from build123d import *
from build123d.topology import SkipClean

# Parameters (mm, degrees)
BOSS_EXTRU_1_START      = -6
BOSS_EXTRU_1_DEPTH      = 6
BOSS_EXTRU_2_START      = -6
BOSS_EXTRU_2_DEPTH      = 2
ENL_V_START             = -4
ESQUISSE3_5_R           = 2.55
ENL_V_MAT_EXTRU_1_DEPTH = 4
ENL_V_START_2           = -16.5
ENL_V_MAT_EXTRU_5_DEPTH = 10.5
CONG_1_R                = 2
CHANFREIN1_SIZE         = 0.5
SYM_TRIE1_START         = -2
SYM_TRIE1_DEPTH         = 10.5
SYM_TRIE1_START_2       = -8
SYM_TRIE1_2_DEPTH       = 4
SYM_TRIE1_START_3       = -7.5000001
SYM_TRIE1_3_DEPTH       = 5.5000001
SYM_TRIE1_START_4       = -4
SYM_TRIE1_4_DEPTH       = 2
SYM_TRIE1_7_DEPTH       = 0.4999999
M3_CLEARANCE_HOLE1_D    = 3.4
BOSS_EXTRU_3_DEPTH      = 8.5
ENL_V_START_3           = -8.5
ENL_V_MAT_EXTRU_2_DEPTH = 8.5
ENL_V_START_4           = -6.5
ESQUISSE5_R             = 1.125
ENL_V_MAT_EXTRU_3_DEPTH = 6
ESQUISSE5_3_R           = 1.125
ENL_V_MAT_EXTRU_4_DEPTH = 6.5
CONG_2_R                = 0.5
CONG_3_R                = 1.5
ENL_V_START_5           = -7.5
ESQUISSE9_R             = 4
ENL_V_MAT_EXTRU_8_DEPTH = 7.5
CONG_5_R                = 1.5


with BuildPart() as part:
    # Esquisse1 → Révolution1 (revolve)
    with BuildSketch(Plane.XY):
        Polygon((-8.5, 8.5), (-6, 8.5), (-6, 0), (-3.5, 0), (-3.5, -1), (-4.383974596, -1), (-5.25, -1.5), (-6.5, -1.5), (-6.5, -6.5), (-6.8, -6.5), (-6.8, -7.2), (-6.5, -7.2), (-6.5, -8), (-8.5, -8), align=None)
    revolve(axis=Axis((0, 6.43509573, 0), (0, -1, 0)))

    # Esquisse3 → Boss.-Extru.1 (add)
    with BuildSketch(Plane.XZ.offset(8).offset(BOSS_EXTRU_1_START)):
        with BuildLine():
            ThreePointArc((-7.928571429, 3.06394437), (-7.728470361, 3.5384666), (-7.5, 4))
            Line((-7.5, 4), (-10.5, 4))
            ThreePointArc((-10.5, 4), (-14.5, 0), (-10.5, -4))
            Line((-10.5, -4), (-7.5, -4))
            ThreePointArc((-7.5, -4), (-7.728470361, -3.5384666), (-7.928571429, -3.06394437))
            ThreePointArc((-7.928571429, -3.06394437), (-8.196108254, -2.252511816), (-8.380833333, -1.418320358))
            ThreePointArc((-8.380833333, -1.418320358), (-13.05, 0), (-8.380833333, 1.418320358))
            ThreePointArc((-8.380833333, 1.418320358), (-8.196108254, 2.252511816), (-7.928571429, 3.06394437))
        make_face()
    extrude(amount=BOSS_EXTRU_1_DEPTH)

    # Esquisse3<4> → Boss.-Extru.2 (add)
    with BuildSketch(Plane.XZ.offset(8).offset(BOSS_EXTRU_2_START)):
        with BuildLine():
            ThreePointArc((-8.380833333, -1.418320358), (-8.5, 0), (-8.380833333, 1.418320358))
            ThreePointArc((-8.380833333, 1.418320358), (-13.05, 0), (-8.380833333, -1.418320358))
        make_face()
    extrude(amount=BOSS_EXTRU_2_DEPTH)

    # Esquisse3<5> → Enlèv. mat.-Extru.1 (cut)
    with BuildSketch(Plane.XZ.offset(8).offset(ENL_V_START)):
        with Locations((-10.5, 0)):
            Circle(ESQUISSE3_5_R)
    extrude(amount=ENL_V_MAT_EXTRU_1_DEPTH, mode=Mode.SUBTRACT)

    # Esquisse3<7> → Enlèv. mat.-Extru.5 (cut)
    with BuildSketch(Plane.XZ.offset(8).offset(ENL_V_START_2)):
        with BuildLine():
            ThreePointArc((-7.5, 4), (-8.5, 0), (-7.5, -4))
            Line((-7.5, -4), (-7.5, 4))
        make_face()
    extrude(amount=ENL_V_MAT_EXTRU_5_DEPTH, mode=Mode.SUBTRACT)

    # Congé1
    cong_1_edges = [part.edges().sort_by_distance(p)[0] for p in [
        (-7.5, -5, 4),
        (-7.5, -5, -4),
    ]]
    fillet(cong_1_edges, radius=CONG_1_R)

    # Chanfrein1
    chanfrein1_edges = [part.edges().sort_by_distance(p)[0] for p in [
        (-8.06008453, -8, 0.741156191),
    ]]
    chamfer(chanfrein1_edges, length=CHANFREIN1_SIZE)

    # Symétrie1: read off the stored shape, not the designer's step
    # Symétrie1 outline → Symétrie1 (cut)
    with BuildSketch(Plane(origin=(0, 0, 0), x_dir=(1, 0, 0), z_dir=(0, 1, 0)).offset(SYM_TRIE1_START)):
        with BuildLine():
            Line((7.5, 4), (7.5, -4))
            ThreePointArc((7.5, -4), (8.5, 0), (7.5, 4))
        make_face()
    extrude(amount=SYM_TRIE1_DEPTH, mode=Mode.SUBTRACT)

    # Sym_trie1 2 outline → Sym_trie1 2 (cut)
    with BuildSketch(Plane(origin=(0, 0, 0), x_dir=(1, 0, 0), z_dir=(0, 1, 0)).offset(SYM_TRIE1_START_2)):
        with BuildLine():
            ThreePointArc((8.380833333, 1.418320358), (7.95, 0), (8.380833333, -1.418320358))
            ThreePointArc((8.380833333, -1.418320358), (8.5, 0), (8.380833333, 1.418320358))
        make_face()
    extrude(amount=SYM_TRIE1_2_DEPTH, mode=Mode.SUBTRACT)

    # Sym_trie1 3 outline → Sym_trie1 3 (add)
    with BuildSketch(Plane(origin=(0, 0, 0), x_dir=(1, 0, 0), z_dir=(0, 1, 0)).offset(SYM_TRIE1_START_3)):
        with BuildLine():
            ThreePointArc((6.975540357, -4.857142857), (7.69102387, -4.227189479), (8.61684397, -4))
            Line((8.61684397, -4), (10.5, -4))
            ThreePointArc((10.5, -4), (14.5, 0), (10.5, 4))
            Line((10.5, 4), (8.61684397, 4))
            ThreePointArc((8.61684397, 4), (7.69102387, 4.227189479), (6.975540357, 4.857142857))
            ThreePointArc((6.975540357, 4.857142857), (7.868349781, 3.215442696), (8.380833333, 1.418320358))
            ThreePointArc((8.380833333, 1.418320358), (13.05, 0), (8.380833333, -1.418320358))
            ThreePointArc((8.380833333, -1.418320358), (7.868349781, -3.215442696), (6.975540357, -4.857142857))
        make_face()
    extrude(amount=SYM_TRIE1_3_DEPTH)

    # Sym_trie1 4 outline → Sym_trie1 4 (add)
    with BuildSketch(Plane(origin=(0, 0, 0), x_dir=(1, 0, 0), z_dir=(0, 1, 0)).offset(SYM_TRIE1_START_4)):
        with BuildLine():
            ThreePointArc((8.380833333, 1.418320358), (8.5, 0), (8.380833333, -1.418320358))
            ThreePointArc((8.380833333, -1.418320358), (13.05, 0), (8.380833333, 1.418320358))
        make_face()
    extrude(amount=SYM_TRIE1_4_DEPTH)

    # Sym_trie1 5 outline → Sym_trie1 5 (revolve, cut)
    with BuildSketch(Plane(origin=(10.5, 0, 0), x_dir=(1, 0, 0), z_dir=(0, 0, 1))):
        Polygon((3.05, -8), (2.55, -7.5), (2.55, -8), align=None)
    revolve(axis=Axis((10.5, 0, 0), (0, 1, 0)), mode=Mode.SUBTRACT)

    # Sym_trie1 6 outline → Sym_trie1 6 (revolve)
    with SkipClean():  # the faces are left unmerged after this step: merging them gives an invalid solid
        with BuildSketch(Plane(origin=(10.5, 0, 0), x_dir=(1, 0, 0), z_dir=(0, 0, 1))):
            Polygon((3.05, -7.5), (2.55, -7.5), (3.05, -8), align=None)
        revolve(axis=Axis((10.5, 0, 0), (0, 1, 0)))

    # Sym_trie1 7 outline → Sym_trie1 7 (add)
    with BuildSketch(Plane(origin=(0, 0, 0), x_dir=(1, 0, 0), z_dir=(0, 1, 0)).offset(SYM_TRIE1_START_2)):
        with BuildLine():
            ThreePointArc((8.2475, 2.056390953), (13.55, 0), (8.2475, -2.056390953))
            ThreePointArc((8.2475, -2.056390953), (7.933495012, -3.051173035), (7.5, -4))
            ThreePointArc((7.5, -4), (7.250447615, -4.436328367), (6.975540357, -4.857142857))
            ThreePointArc((6.975540357, -4.857142857), (7.69102387, -4.227189479), (8.61684397, -4))
            Line((8.61684397, -4), (10.5, -4))
            ThreePointArc((10.5, -4), (14.5, 0), (10.5, 4))
            Line((10.5, 4), (8.61684397, 4))
            ThreePointArc((8.61684397, 4), (7.69102387, 4.227189479), (6.975540357, 4.857142857))
            ThreePointArc((6.975540357, 4.857142857), (7.250447615, 4.436328367), (7.5, 4))
            ThreePointArc((7.5, 4), (7.933495012, 3.051173035), (8.2475, 2.056390953))
        make_face()
    extrude(amount=SYM_TRIE1_7_DEPTH)

    # M3 Clearance Hole1 (through all)
    with Locations(Plane(origin=(0, -4, 0), x_dir=(-1, 0, 0), z_dir=(0, -1, 0))):
        with Locations((10.5, 0), (-10.5, 0)):
            Hole(M3_CLEARANCE_HOLE1_D / 2)

    # Esquisse4 → Boss.-Extru.3 (add)
    with BuildSketch(Plane(origin=(0, 8.5, 0), x_dir=(1, 0, 0), z_dir=(0, 1, 0))):
        with BuildLine():
            Line((7.5, 14.5), (-7.5, 14.5))
            Line((-7.5, 14.5), (-7.5, 4))
            ThreePointArc((-7.5, 4), (-1.593272922, 8.349340177), (5.5, 6.480740698))
            Line((5.5, 6.480740698), (5.5, 13))
            Line((5.5, 13), (6, 13))
            Line((6, 13), (6, 6.020797289))
            ThreePointArc((6, 6.020797289), (6.825203691, 5.066220937), (7.5, 4))
            Line((7.5, 4), (7.5, 14.5))
        make_face()
    extrude(amount=-BOSS_EXTRU_3_DEPTH)

    # Esquisse4<3> → Enlèv. mat.-Extru.2 (cut)
    with BuildSketch(Plane(origin=(0, 8.5, 0), x_dir=(1, 0, 0), z_dir=(0, 1, 0)).offset(ENL_V_START_3)):
        with BuildLine():
            Line((6, 0), (6, 13))
            Line((6, 13), (5.5, 13))
            Line((5.5, 13), (5.5, 2.397915762))
            ThreePointArc((5.5, 2.397915762), (5.873670062, 1.224744871), (6, 0))
        make_face()
    extrude(amount=ENL_V_MAT_EXTRU_2_DEPTH, mode=Mode.SUBTRACT)

    # Esquisse5 → Enlèv. mat.-Extru.3 (cut)
    with BuildSketch(Plane(origin=(7.5, 0, 0), x_dir=(0, 0, -1), z_dir=(1, 0, 0)).offset(ENL_V_START_4)):
        with Locations((9.875, 4.2554)):
            Circle(ESQUISSE5_R)
        with BuildLine():
            Line((8.75, 8.5), (8.75, 4.2554))
            ThreePointArc((8.75, 4.2554), (9.875, 5.3804), (11, 4.2554))
            Line((11, 4.2554), (11, 8.5))
            Line((11, 8.5), (8.75, 8.5))
        make_face()
    extrude(amount=-ENL_V_MAT_EXTRU_3_DEPTH, mode=Mode.SUBTRACT)

    # Esquisse5<3> → Enlèv. mat.-Extru.4 (cut)
    with BuildSketch(Plane(origin=(7.5, 0, 0), x_dir=(0, 0, -1), z_dir=(1, 0, 0))):
        with Locations(Location((9.875, 4.2554, 0), (0, 0, 180))):
            Circle(ESQUISSE5_3_R)
    extrude(amount=-ENL_V_MAT_EXTRU_4_DEPTH, mode=Mode.SUBTRACT)

    # Congé2
    # the kernel refuses this fillet: 0.5 mm, written as the material it takes off along each edge
    with BuildSketch(Plane(origin=(5.5, 0, -2.397915762), x_dir=(0, 0, -1), z_dir=(0, 1, 0))) as cong_2_piece_1:
        with BuildLine():
            CenterArc((1.75539617, 0.5), CONG_2_R, 129.715137232, 140.284862768)
            ThreePointArc((1.435910637, 0.884615385), (0.749192225, 0.391603841), (0, 0))
            Line((0, 0), (1.75539617, 0))
        make_face()
    extrude(amount=12.888490425, mode=Mode.SUBTRACT)

    # Congé3
    cong_3_edges = [part.edges().sort_by_distance(p)[0] for p in [
        (7.5, 3.25, 4),
        (7.5, 4.25, -14.5),
        (-7.5, 4.25, -14.5),
        (-7.5, 3.25, 4),
    ]]
    fillet(cong_3_edges, radius=CONG_3_R)

    # Esquisse9 → Enlèv. mat.-Extru.8 (cut)
    with BuildSketch(Plane(origin=(0, 8.5, 0), x_dir=(1, 0, 0), z_dir=(0, 1, 0)).offset(ENL_V_START_5)):
        with Locations((-10.5, 0)):
            Circle(ESQUISSE9_R)
        with Locations((10.5, 0)):
            Circle(ESQUISSE9_R)
    extrude(amount=ENL_V_MAT_EXTRU_8_DEPTH, mode=Mode.SUBTRACT)

    # Congé5
    cong_5_edges = [part.edges().sort_by_distance(p)[0] for p in [
        (7.5, 4.75, -2.645751311),
        (7.5, 4.75, 2.645751311),
        (-7.5, 4.75, -2.645751311),
        (-7.5, 4.75, 2.645751311),
    ]]
    fillet(cong_5_edges, radius=CONG_5_R)


solid = part.part
Read the model definition and answer for the solid it produces. Units are mm, in the model's axes. A direction names the side the tool comes from. Give positions to 0.01 mm unless a question says otherwise; leave off trailing zeros. Loops run counter-clockwise (first coordinate to the right, second up) from the corner with the lowest first, then second, coordinate; pieces in that order, holes last. Notation, with made-up numbers: M -6,84 L 25,84 A17 ccw 25,104 Z; hole C -6.75,14 d5. An arc over 180 degrees is marked long. Write each question's results on one line, items separated by ' | '.
1. Given pin 1 (0.6 mm diameter, centred on x = -9.5, y = -4, fed in from -Z); pin 2 (2.5 mm diameter, centred on y = 6.5, z = -10, fed in from -X); pin 3 (1.3 mm diameter, centred on y = 4.26, z = -9.88, fed in from +X); pin 4 (1.5 mm diameter, centred on y = -2.5, z = -10.5, fed in from +X), each flat-ended and moving along its own axis, determine where each tip first touches the part or whether it passes through.
Values:
pin 1: stops at z = -4 | pin 2: stops at x = -7.5 | pin 3: stops at x = -5 | pin 4: passes through
2. The mould has two halves that part along Z. Classify faces 6 (the face through (7, 1, 0)), 7 (the face through (-14.5, -5, 0.1)), 8 (the face through (0, 0, -10)): pulls with the +Z half, pulls with the -Z half, needs draft (parallel to the pull), parting line crosses it, or undercut.
Values:
face 6: undercut | face 7: parting line crosses it | face 8: needs draft
3. Section A-A on y = -2.5 is taken. Give the vertices of the cut face in (x, z), plus the area to 3 significant figures.
Values:
outline: M -10.5,-4 L -8.62,-4 A2 cw -6.98,-4.86 A8.5 ccw 6.98,-4.86 A2 cw 8.62,-4 L 10.5,-4 A4 ccw 10.5,4 L 8.62,4 A2 cw 6.98,4.86 A8.5 ccw -6.98,4.86 A2 cw -8.62,4 L -10.5,4 A4 ccw Z; hole C -10.5,0 d3.4; hole C 0,0 d13; hole C 10.5,0 d3.4 | area: 164 mm^2
4. A tool of negligible diameter and unlimited length cuts with its end or side. For faces 1 (the face through (-7.703, -5.042, -4.221)), 2 (the face through (5.16, 4.19, -3.68)), 3 (the face through (6.5, 4.7, 0)), 4 (the face through (5.158, -4.035, 3.955)), 5 (the face through (-7.5, 3, -7)), from which of +Z, -Z, +X, -X, +Y, -Y can it reach the whole face along a straight path? Write none if from no direction.
Values:
face 1: -Z, -X, -Y | face 2: +Y | face 3: +X, +Y | face 4: -Y | face 5: +Z, -Z, -X, +Y
5. Straight lines are drawn through the part: line 1 (X direction, y = -4.95, z = 0); line 2 (X direction, y = -6.65, z = 0); line 3 (Z direction, x = 0, y = 6). For each, find the intervals that lie inside material, in ascending order. Write a range as [from, to].
Values:
line 1: x = [-14.5, -13.05], [-7.95, -6.5], [6.5, 7.95], [13.05, 14.5] | line 2: x = [-14.5, -13.05], [-7.95, -6.8], [6.8, 7.95], [13.05, 14.5] | line 3: z = [-14.5, -11], [-8.75, -6], [6, 8.5]
